from build123d import *

# Parameters (mm, degrees)
ESQUISSE1_W             = 35
ESQUISSE1_H             = 35
BOSS_EXTRU_1_DEPTH      = 5
BOSS_EXTRU_2_DEPTH      = 13.13
ESQUISSE3_W             = 5
ESQUISSE3_H             = 35
BOSS_EXTRU_3_DEPTH      = 5
BOSS_EXTRU_4_START      = -19.05
ESQUISSE4_W             = 20.5
ESQUISSE4_H             = 4.65
BOSS_EXTRU_4_DEPTH      = 5
BOSS_EXTRU_5_START      = 27.4
ESQUISSE5_W             = 5
ESQUISSE5_H             = 20.5
BOSS_EXTRU_5_DEPTH      = 5
BOSS_EXTRU_6_START      = -1.1625
BOSS_EXTRU_6_DEPTH      = 2.325
BOSS_EXTRU_7_START      = 27.225
BOSS_EXTRU_7_DEPTH      = 2.325
CONG_3_R                = 5
CONG_4_R                = 1.3
CONG_5_R                = 5
ESQUISSE8_R             = 1
ENL_V_MAT_EXTRU_1_DEPTH = 38.415270946
CHANFREIN1_SIZE         = 1.5
CONG_6_R                = 5
CONG_7_R                = 2.5
CONG_8_R                = 2.5
CONG_9_R                = 2.5
ESQUISSE9_R             = 1.5
ENL_V_MAT_EXTRU_2_DEPTH = 51.326434406


# Some blends are built 0.0001 mm under size
with BuildPart() as part:
    # Esquisse1 → Boss.-Extru.1 (new body)
    with BuildSketch(Plane.XY):
        Rectangle(ESQUISSE1_W, ESQUISSE1_H)
    extrude(amount=BOSS_EXTRU_1_DEPTH)

    # Esquisse2 → Boss.-Extru.2 (add)
    with BuildSketch(Plane(origin=(0, 0, 0), x_dir=(-1, 0, 0), z_dir=(0, 0, -1))):
        Polygon((25, 15), (25, -15), (25, -17.5), (27.5, -17.5), (27.5, 17.5), (25, 17.5), align=None)
        Polygon((17.5, 17.5), (17.5, -17.5), (20, -17.5), (20, -15), (20, 15), (20, 17.5), align=None)
    extrude(amount=-BOSS_EXTRU_2_DEPTH)


with BuildPart() as boss_extru_2_piece_1:
    # of the separate pieces the step leaves, piece 1, a body of its own (boss_extru_2_pieces)
    add(part.part.solids().sort_by_distance((17.5, 17.5, 0))[0])



with BuildPart() as boss_extru_2_piece_2:
    # of the separate pieces the step leaves, piece 2, a body of its own (boss_extru_2_pieces)
    add(part.part.solids().sort_by_distance((-25, 17.5, 0))[0])


with BuildPart() as boss_extru_2_piece_1_1:
    add(boss_extru_2_piece_1.part)

    add(boss_extru_2_piece_2.part)  # Boss.-Extru.3 merges Boss.-Extru.2 piece 2
    # Esquisse3 → Boss.-Extru.3 (add)
    with BuildSketch(Plane.ZY.offset(20)):
        with Locations((10.63, 0)):
            Rectangle(ESQUISSE3_W, ESQUISSE3_H)
    extrude(amount=BOSS_EXTRU_3_DEPTH)

    # Esquisse4 → Boss.-Extru.4 (add)
    with BuildSketch(Plane.ZY.offset(27.5).offset(BOSS_EXTRU_4_START)):
        with Locations((-10.25, -15.175)):
            Rectangle(ESQUISSE4_W, ESQUISSE4_H)
    extrude(amount=BOSS_EXTRU_4_DEPTH)

    # Esquisse5 → Boss.-Extru.5 (add)
    with BuildSketch(Plane(origin=(0, -12.85, 0), x_dir=(1, 0, 0), z_dir=(0, 1, 0)).offset(BOSS_EXTRU_5_START)):
        with Locations((-10.95, 10.25)):
            Rectangle(ESQUISSE5_W, ESQUISSE5_H)
    extrude(amount=-BOSS_EXTRU_5_DEPTH)

    # Esquisse6 → Boss.-Extru.6 (add)
    with BuildSketch(Plane.XZ.offset(17.5).offset(BOSS_EXTRU_6_START)):
        Polygon((-8.45, -8), (4.23857754, 0), (-8.45, 0), align=None)
    extrude(amount=-BOSS_EXTRU_6_DEPTH)

    # Esquisse7 → Boss.-Extru.7 (add)
    with BuildSketch(Plane(origin=(0, -14.0125, 0), x_dir=(1, 0, 0), z_dir=(0, 1, 0)).offset(BOSS_EXTRU_7_START)):
        Polygon((-8.45, 8), (-8.45, 0), (4.23857754, 0), align=None)
    extrude(amount=-BOSS_EXTRU_7_DEPTH)

    # Congé3
    # the kernel refuses this fillet: 5 mm, written as the material it adds along each edge
    with BuildSketch(Plane(origin=(12.251689354, -16.3375, 0), x_dir=(0, -1, 0), z_dir=(-1, 0, 0))) as cong_3_piece_1_section:
        with BuildLine():
            CenterArc((5, -3.205244725), CONG_3_R, 140.129918766, 39.870081234)
            Line((0, -3.205244725), (0, 0))
            Line((0, 0), (1.1625, 0))
        make_face()
    cong_3_piece_1 = extrude(amount=20.701689354, mode=Mode.PRIVATE)
    cong_3_piece_1 = split(cong_3_piece_1, bisect_by=Plane(origin=(-0.976512405, -16.627700283, -3.288053324), z_dir=(-0.5333333333333334, 0, 0.8459051693633013)), keep=Keep.TOP, mode=Mode.PRIVATE)
    add(cong_3_piece_1)

    # Congé4
    cong_4_edges = [boss_extru_2_piece_1_1.edges().sort_by_distance(p)[0] for p in [
        (-2.10571123, 13.2125, 0),
    ]]
    fillet(cong_4_edges, radius=CONG_4_R)

    # Congé5
    cong_5_edges = [boss_extru_2_piece_1_1.edges().sort_by_distance(p)[0] for p in [
        (17.5, -17.5, 2.5),
        (17.5, 17.5, 2.5),
    ]]
    fillet(cong_5_edges, radius=CONG_5_R)

    # Esquisse8 → Enlèv. mat.-Extru.1 (cut, through all)
    with BuildSketch(Plane(origin=(-8.45, 0, 0), x_dir=(0, 0, -1), z_dir=(1, 0, 0))):
        with Locations(Location((14.4, 12.225, 0), (0, 0, 90))):
            Circle(ESQUISSE8_R)
        with Locations(Location((14.4, -15.175, 0), (0, 0, 90))):
            Circle(ESQUISSE8_R)
    extrude(amount=-ENL_V_MAT_EXTRU_1_DEPTH, mode=Mode.SUBTRACT)

    # Chanfrein1
    chanfrein1_edges = [boss_extru_2_piece_1_1.edges().sort_by_distance(p)[0] for p in [
        (-10.95, -12.85, -20.5),
        (-10.95, -17.5, -20.5),
        (-10.95, 9.55, -20.5),
        (-10.95, 14.55, -20.5),
    ]]
    chamfer(chanfrein1_edges, length=CHANFREIN1_SIZE)

    # Congé6
    cong_6_edges = [boss_extru_2_piece_1_1.edges().sort_by_distance(p)[0] for p in [
        (-10.95, -12.85, 0),
        (-10.95, 9.55, 0),
    ]]
    fillet(cong_6_edges, radius=CONG_6_R)

    # Congé7
    cong_7_edges = [boss_extru_2_piece_1_1.edges().sort_by_distance(p)[0] for p in [
        (-17.5, 0, 13.13),
        (-27.5, 0, 13.13),
    ]]
    fillet(cong_7_edges, radius=CONG_7_R)

    # Congé8
    cong_8_edges = [boss_extru_2_piece_1_1.edges().sort_by_distance(p)[0] for p in [
        (-17.5, 0, 5),
    ]]
    fillet(cong_8_edges, radius=CONG_8_R)

    # Congé9
    cong_9_edges = [boss_extru_2_piece_1_1.edges().sort_by_distance(p)[0] for p in [
        (-20, 0, 0),
        (-25, 0, 0),
    ]]
    fillet(cong_9_edges, radius=CONG_9_R - 0.0001)  # a hair under: the kernel refuses the full size

    # Esquisse9 → Enlèv. mat.-Extru.2 (cut, through all)
    with BuildSketch(Plane(origin=(-25, 0, 0), x_dir=(0, 0, -1), z_dir=(1, 0, 0))):
        with Locations((-5.315, -12)):
            Circle(ESQUISSE9_R)
        with Locations((-5.315, 12)):
            Circle(ESQUISSE9_R)
    extrude(amount=-ENL_V_MAT_EXTRU_2_DEPTH, mode=Mode.SUBTRACT)


solid = boss_extru_2_piece_1_1.part
Here's how the part is built. I have some questions about the finished solid (model axes, mm). A direction names the side the tool comes from. Coordinates: 2 decimals unless noted, no trailing zeros. Loops run counter-clockwise (first coordinate to the right, second up) from the corner with the lowest first, then second, coordinate; pieces in that order, holes last. Notation, with made-up numbers: (43, -4) -> (53, -4) arc R34 cw to (53, 31) -> close; hole circle Ø4 at (15.25, -1.5). An arc over 180 degrees is marked (long way). Use one line per item in the form item = value. Start each with the question number.
(1) Please list where these lines run through material, in increasing order: line 1 along X through (y, z) = (-14, -8); line 2 along Z through (x, y) = (2, -3.5); line 3 along X through (y, z) = (-3, 4).
(2) If we section it at C-C (x = -3): Please give me the cut outline in (y, z), then the cut area to 3 significant figures.
(3) On a 3-axis mill with a long thin cutter (end or side, diameter ignored), from which of +Z, -Z, +X, -X, +Y, -Y can I reach the whole of each face in a straight line? I mean faces 1 (the face through (-13.45, -15, -10)), 2 (the face through (-19.248, 0.245, 0.713)), 3 (the face through (-17.5, 0, 9)), 4 (the face through (-26.232, 12.066, 6.814)). Say none if no direction works.
(4) Will these pins go through, and if not, where does the flat tip stop? pin 1 (2.5 mm diameter, centred on x = -11, z = -12.5, fed in from +Y); pin 2 (3.5 mm diameter, centred on y = 1.5, z = 8.5, fed in from +X); pin 3 (4 mm diameter, centred on x = -3.5, y = 0, fed in from +Z).
(5) If we section it at A-A (z = -14.4): Please give me the cut outline in (x, y) (3 decimals).
(6) If we section it at D-D (z = -2.5): Please give me the cut outline in (x, y).
(7) We'd pull the mould along X, two halves only. Please class faces 5 (the face through (-25, 0, 5)), 6 (the face through (-11, -12.85, -12)), 7 (the face through (-18.213, -0.245, 12.378)): pulls with the +X half, pulls with the -X half, needs draft (parallel to the pull), parting line crosses it, or undercut.
Verdict:
q1.line_1 = -13.45 to -8.45
q1.line_2 = 0 to 5
q1.line_3 = -27.5 to -25, -20 to 17.5
q2.outline = (-17.5, 0) arc R5 cw to (-16.34, -3.21) -> (-16.34, -4.56) -> (-14.01, -4.56) -> (-14.01, 0) -> (10.89, 0) -> (10.89, -4.56) -> (13.21, -4.56) -> (13.21, -1.3) arc R1.3 cw to (14.51, 0) -> (17.5, 0) -> (17.5, 5) -> (-17.5, 5) -> close
q2.area = 198 mm²
q3.face_1 = -Z, -X, +Y, -Y
q3.face_2 = -Z, +Y, -Y
q3.face_3 = +Z, +X, +Y, -Y
q3.face_4 = -X
q4.pin_1 = 14.55
q4.pin_2 = -17.38
q4.pin_3 = 5
q5.outline = (-13.45, -17.5) -> (-8.45, -17.5) -> (-8.45, -16.175) -> (-13.45, -16.175) -> close; (-13.45, -14.175) -> (-8.45, -14.175) -> (-8.45, -12.85) -> (-13.45, -12.85) -> close; (-13.45, 9.55) -> (-8.45, 9.55) -> (-8.45, 11.225) -> (-13.45, 11.225) -> close; (-13.45, 13.225) -> (-8.45, 13.225) -> (-8.45, 14.55) -> (-13.45, 14.55) -> close
q6.outline = (-13.45, -17.5) -> (-8.45, -17.5) -> (-8.45, -16.39) -> (0.27, -16.39) -> (0.27, -14.01) -> (-8.45, -14.01) -> (-8.45, -12.18) -> (-13.45, -12.18) -> close; (-13.45, 8.88) -> (-8.45, 8.88) -> (-8.45, 10.89) -> (0.27, 10.89) -> (0.27, 13.21) -> (-8.45, 13.21) -> (-8.45, 14.55) -> (-13.45, 14.55) -> close
q7.face_5 = undercut
q7.face_6 = needs draft
q7.face_7 = pulls with the +X half
